Design review of the part built by this model. Coordinates are the model's own, in mm. Face numbers are marked on the shaded views. A direction names the side the tool comes from. Coordinates: 2 decimals unless noted, no trailing zeros. Write each loop counter-clockwise with the first axis right and the second up, starting at its lowest first coordinate (ties: lowest second). Pieces come first, ordered by that corner, then holes. Notation, with made-up numbers: (13.5, 16) - (20.5, 16) arc R21 ccw to (20.5, 29) - close; hole circle Ø10 at (52, 47). An arc over 180 degrees is marked (long way). One line per item, written item: value.
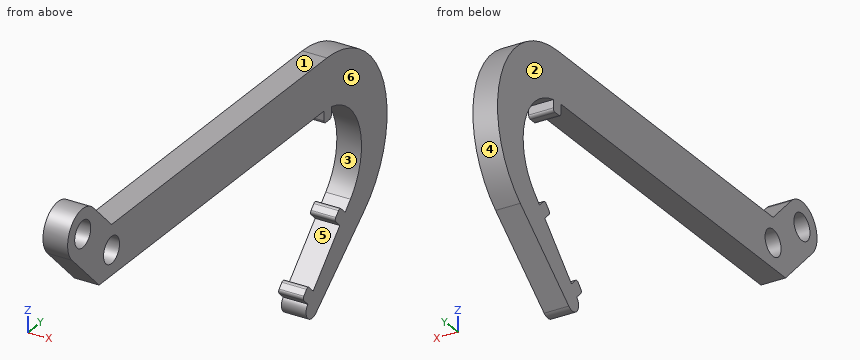
from build123d import *

# Parameters (mm, degrees)
BOSS_EXTRUDE1_DEPTH         = 6.35
F_1_4_CLEARANCE_HOLE1_D     = 6.7564
F_1_4_CLEARANCE_HOLE1_DEPTH = 8.382
F_1_4_CLEARANCE_HOLE1_TIP   = 2.029827343
BOSS_EXTRUDE2_DEPTH         = 6.35
CRVPATTERN2_START           = 12.7
CRVPATTERN2_OUTLINE_W       = 6.35
CRVPATTERN2_OUTLINE_H       = 3.175
CRVPATTERN2_DEPTH           = 3.175
SKETCH5_W                   = 3.175
SKETCH5_H                   = 3.175
BOSS_EXTRUDE3_DEPTH         = 6.35
FILLET1_R                   = 0.762


# Read off the part's stored shape, not the designer's step: CrvPattern2
with BuildPart() as part:
    # Sketch1 → Boss-Extrude1 (new body)
    with BuildSketch(Plane(origin=(0, 0, 0), x_dir=(0, 0, -1), z_dir=(1, 0, 0))):
        with BuildLine():
            Line((-28.575, -89.444743879), (-28.575, 1.27))
            ThreePointArc((-28.575, 1.27), (-11.551976139, 25.24887134), (16.699509509, 17.086569533))
            Line((16.699509509, 17.086569533), (32.969334569, -3.357483913))
            ThreePointArc((32.969334569, -3.357483913), (32.673446977, -6.833926713), (29.185832393, -6.735192091))
            Line((29.185832393, -6.735192091), (11.225320151, 11.225320151))
            ThreePointArc((11.225320151, 11.225320151), (-6.075099489, 14.666587579), (-15.875, 0))
            Line((-15.875, 0), (-15.875, -94.705256121))
            Line((-15.875, -94.705256121), (-27.259871939, -106.090128061))
            ThreePointArc((-27.259871939, -106.090128061), (-36.240128061, -106.090128061), (-36.240128061, -97.109871939))
            Line((-36.240128061, -97.109871939), (-28.575, -89.444743879))
        make_face()
    extrude(amount=BOSS_EXTRUDE1_DEPTH)

    # 1/4 Clearance Hole1
    with Locations(Plane(origin=(6.35, 0, 0), x_dir=(0, 0, -1), z_dir=(1, 0, 0))):
        with Locations((-22.225, -89.444743879), (-31.75, -101.6)):
            Hole(F_1_4_CLEARANCE_HOLE1_D / 2, depth=F_1_4_CLEARANCE_HOLE1_DEPTH)
            with Locations((0, 0, -(F_1_4_CLEARANCE_HOLE1_DEPTH + F_1_4_CLEARANCE_HOLE1_TIP / 2))):  # 118° drill point
                Cone(0, F_1_4_CLEARANCE_HOLE1_D / 2, F_1_4_CLEARANCE_HOLE1_TIP, mode=Mode.SUBTRACT)

    # Sketch4 → Boss-Extrude2 (add)
    with BuildSketch(Plane(origin=(6.35, 0, 0), x_dir=(0, 0, -1), z_dir=(1, 0, 0))):
        Polygon((29.185832393, -6.735192091), (26.940768363, -8.980256121), (24.695704333, -6.735192091), (26.940768363, -4.490128061), align=None)
    extrude(amount=-BOSS_EXTRUDE2_DEPTH)

    # CrvPattern2 outline → CrvPattern2 (add)
    with BuildSketch(Plane(origin=(0, 0, 0), x_dir=(1, 0, 0), z_dir=(0, 0.7071067811865476, -0.7071067811865476)).offset(CRVPATTERN2_START)):
        with Locations((3.175, 4.7625)):
            Rectangle(CRVPATTERN2_OUTLINE_W, CRVPATTERN2_OUTLINE_H)
    extrude(amount=CRVPATTERN2_DEPTH)

    # Sketch5 → Boss-Extrude3 (add)
    with BuildSketch(Plane(origin=(6.35, 0, 0), x_dir=(0, 0, -1), z_dir=(1, 0, 0))):
        with Locations((-14.2875, 1.5875)):
            Rectangle(SKETCH5_W, SKETCH5_H)
    extrude(amount=-BOSS_EXTRUDE3_DEPTH)

    # Fillet1
    fillet1_edges = [part.edges().sort_by_distance(p)[0] for p in [
        (3.175, 4.490128061, -13.470384182),
        (3.175, 6.735192091, -11.225320151),
        (3.175, 3.175, 12.7),
        (3.175, 0, 12.7),
        (3.175, -8.980256121, -26.940768363),
        (3.175, -6.735192091, -24.695704333),
    ]]
    fillet(fillet1_edges, radius=FILLET1_R)


solid = part.part
1. Consider section C-C, the plane z = 31.75. Write out the cut boundary in (x, y), then the cut area to 3 significant figures.
Answer block:
outline: (0, -107.95) - (6.35, -107.95) - (6.35, -104.98) - (0, -104.98) - close; (0, -98.22) - (6.35, -98.22) - (6.35, -92.62) - (0, -92.62) - close
area: 54.4 mm^2
2. Mouldability with a two-part tool opening along Y and no side actions: class the marked faces 3, 4, 5 and 6 as released by +Y, released by -Y, zero draft, split by the parting line, or undercut.
Answer block:
face 3: undercut
face 4: released by +Y
face 5: undercut
face 6: zero draft
3. Wall thickness on line 1 along Z through (x, y) = (1, -16) (3 decimals); line 2 along Y through (x, z) = (5.5, 33); line 3 along Y through (x, z) = (4, 31.75): over which ranges is each line inside the solid? List them lowest first.
Answer block:
line 1: z = 15.875 to 28.575
line 2: y = -107.83 to -104.74, -98.46 to -93.87
line 3: y = -107.95 to -104.98, -98.22 to -92.62
4. Consider section B-B, the plane x = 3.25. Give the number of separate pieces and of enclosed holes in the cut face, then the cut area to 3 significant figures.
Answer block:
separate pieces: 1
enclosed holes: 2
area: 2,110 mm^2
5. Consider section A-A, the plane y = -101.6. Write out the cut boundary in (x, z), then the cut area to 3 significant figures.
Answer block:
outline: (0, 22.77) - (6.35, 22.77) - (6.35, 28.37) - (0, 28.37) - close; (0, 35.13) - (6.35, 35.13) - (6.35, 38.1) - (0, 38.1) - close
area: 54.4 mm^2
6. For the marked faces 1 and 2, list the 3-axis set-ups (+Z, -Z, +X, -X, +Y, -Y) from which the entire face can be reached by the end or side of a thin tool; tool diameter is ignored.
Answer block:
face 1: +Z, +X, -X, +Y
face 2: +Z, -Z, -X, +Y, -Y
7. Consider section D-D, the plane y = -16. Write out the cut boundary in (x, z) (3 decimals).
Answer block:
outline: (0, 15.875) - (6.35, 15.875) - (6.35, 28.575) - (0, 28.575) - close
8. Insertion check: pin 1 Ø2 at (x, y) = (1.5, -40.5) entering from -Z (3 decimals); pin 2 Ø0.8 at (x, y) = (3, 1.5) entering from -Z; pin 3 Ø2.5 at (x, z) = (2, 15) entering from +Y; pin 4 Ø11 at (y, z) = (-89.44, 22.22) entering from +X. Each pin has a flat end and moves straight along its axis. Give the tip position at first contact, or say it passes through.
Answer block:
pin 1: stops at z = 15.875
pin 2: stops at z = -29.42
pin 3: stops at y = 24.36
pin 4: stops at x = 6.35
